Here's the drawing with two shaded views (mm, measured from the low corner). I have some questions. Round coordinates to 2 decimals unless told otherwise and drop trailing zeros. Order: outer loops, then holes, each group sorted by start corner. A loop starts at its lowest first (then second) coordinate and runs counter-clockwise, first axis right, second up. Notation, with made-up numbers: (70, 89.25) -> (101, 89.25) arc R30 cw to (101, 112.25) -> close; hole circle Ø7 at (37.5, -27.75). An arc over 180 degrees is marked (long way). Answer in a Markdown table with one row per item.
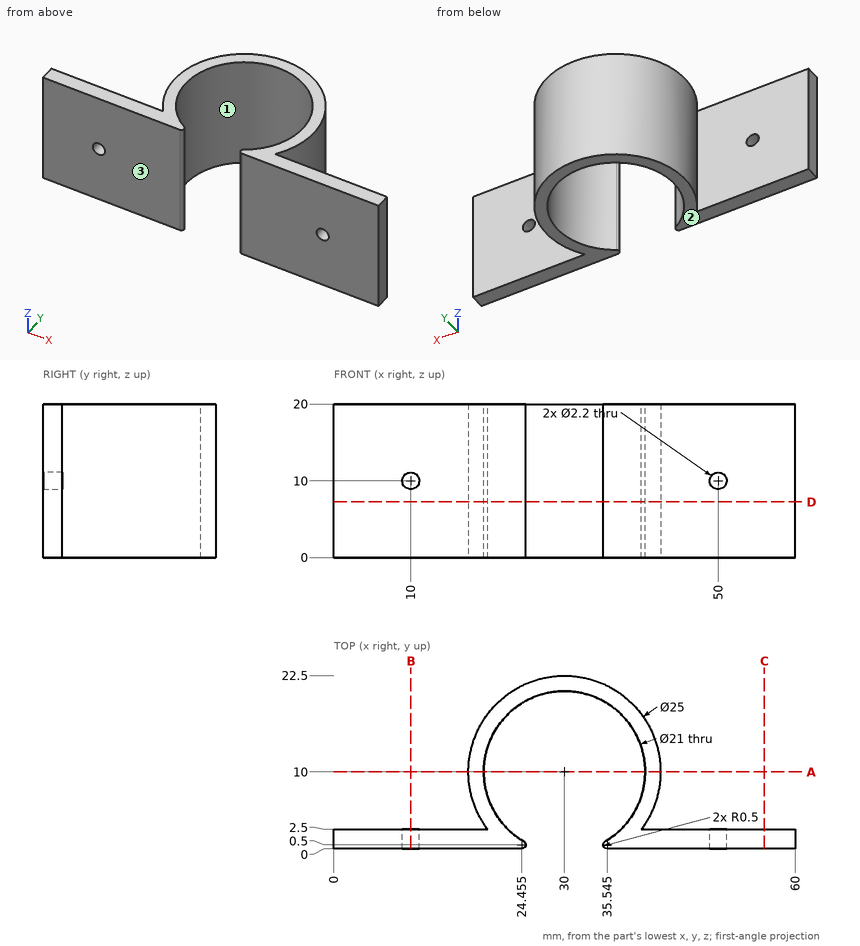
1. Suppose I cut it at A-A on y = 10. Write out the boundary of the cut face in (x, z), then the cut area to 3 significant figures.
Numbers:
| item | result |
|---|---|
| outline | (17.5, 0) -> (19.5, 0) -> (19.5, 20) -> (17.5, 20) -> close; (40.5, 0) -> (42.5, 0) -> (42.5, 20) -> (40.5, 20) -> close |
| area | 80.0 mm2 |
2. Suppose I cut it at C-C on x = 56. Write out the boundary of the cut face in (y, z).
Numbers:
| item | result |
|---|---|
| outline | (0, 0) -> (2.5, 0) -> (2.5, 20) -> (0, 20) -> close |
3. For pin 1 Ø6 at (y, z) = (14.5, 15.5) entering from +X; pin 2 Ø10 at (x, z) = (13.5, 10.5) entering from +Y; pin 3 Ø3 at (y, z) = (9.5, 17) entering from +X, each with a flat end and sliding along its axis, tell me the tip position at first contact or that it passes through.
Numbers:
| item | result |
|---|---|
| pin 1 | stops at x = 42.41 |
| pin 2 | stops at y = 14.9 |
| pin 3 | stops at x = 42.5 |
4. We'd pull the mould along Y, two halves only. Please class the marked faces 1, 2 and 3: released by +Y, released by -Y, zero draft, split by the parting line, or undercut.
Numbers:
| item | result |
|---|---|
| face 1 | undercut |
| face 2 | zero draft |
| face 3 | released by -Y |
5. Please list where these lines run through material, in increasing order: line 1 along Z through (x, y) = (50, 1.2); line 2 along X through (y, z) = (1.65, 10) (1 decimal); line 3 along X through (y, z) = (1.3, 10).
Numbers:
| item | result |
|---|---|
| line 1 | z = 0 to 8.9, 11.1 to 20 |
| line 2 | x = 0 to 8.9, 11.1 to 23.6, 36.4 to 48.9, 51.1 to 60 |
| line 3 | x = 0 to 8.9, 11.1 to 24.12, 35.88 to 48.9, 51.1 to 60 |
6. Suppose I cut it at D-D on z = 7.25. Write out the boundary of the cut face in (x, y) (1 decimal).
Numbers:
| item | result |
|---|---|
| outline | (0, 0) -> (24.5, 0) arc R0.5 ccw to (24.7, 0.9) arc R10.5 cw (long way) to (35.3, 0.9) arc R0.5 ccw to (35.5, 0) -> (60, 0) -> (60, 2.5) -> (40, 2.5) arc R12.5 ccw (long way) to (20, 2.5) -> (0, 2.5) -> close |
7. Suppose I cut it at B-B on x = 10. Write out the boundary of the cut face in (y, z), then the cut area to 3 significant figures.
Numbers:
| item | result |
|---|---|
| outline | (0, 0) -> (2.5, 0) -> (2.5, 8.9) -> (0, 8.9) -> close; (0, 11.1) -> (2.5, 11.1) -> (2.5, 20) -> (0, 20) -> close |
| area | 44.5 mm2 |
